Can you work these out from the model? Positions are in its coordinate system, mm. A direction names the side the tool comes from. Round coordinates to 2 decimals unless told otherwise and drop trailing zeros. Loops run counter-clockwise (first coordinate to the right, second up) from the corner with the lowest first, then second, coordinate; pieces in that order, holes last. Notation, with made-up numbers: (-34.5, 82) -> (-14.5, 82) arc R17 ccw to (-14.5, 88) -> close; hole circle Ø4 at (-4.75, 8). An arc over 180 degrees is marked (long way). Use a Markdown table: item, result.
from build123d import *

# Parameters (mm, degrees)
SKETCH_1_R          = 2.5
EXTRUDE_1_DEPTH     = 180
SKETCH_2_R          = 82.250528809
CUT_EXTRUDE_1_DEPTH = 10
SKETCH_3_R          = 47.359827943
CUT_EXTRUDE_2_DEPTH = 200
SKETCH_4_R          = 50.055938799
CUT_EXTRUDE_3_DEPTH = 30
SKETCH_5_R          = 35.776746529
CUT_EXTRUDE_4_DEPTH = 40
SKETCH_1_3_R        = 2.5
EXTRUDE_2_DEPTH     = 200
SKETCH_6_R          = 45.508426161
CUT_EXTRUDE_5_DEPTH = 50
SKETCH_7_R          = 85.251485325
CUT_EXTRUDE_7_DEPTH = 20


with BuildPart() as part:
    # Sketch 1 → Extrude 1 (new, symmetric)
    with BuildSketch(Plane(origin=(0, 0, 0), x_dir=(1, 0, 0), z_dir=(0, 1, 0))):
        Polygon((-15, -3.15), (-12.5, -3.15), (-12.5, -5.15), (-7, -5.15), (-7, -3.15), (-4.5, -3.15), (-4.5, 3.15), (-7, 3.15), (-7, 5.15), (-12.5, 5.15), (-12.5, 3.15), (-15, 3.15), (-15, 15), (-3.15, 15), (-3.15, 12.5), (-5.15, 12.5), (-5.15, 7), (-3.15, 7), (-3.15, 4.5), (3.15, 4.5), (3.15, 7), (5.15, 7), (5.15, 12.5), (3.15, 12.5), (3.15, 15), (15, 15), (15, 3.15), (12.5, 3.15), (12.5, 5.15), (7, 5.15), (7, 3.15), (4.5, 3.15), (4.5, -3.15), (7, -3.15), (7, -5.15), (12.5, -5.15), (12.5, -3.15), (15, -3.15), (15, -15), (3.15, -15), (3.15, -12.5), (5.15, -12.5), (5.15, -7), (3.15, -7), (3.15, -4.5), (-3.15, -4.5), (-3.15, -7), (-5.15, -7), (-5.15, -12.5), (-3.15, -12.5), (-3.15, -15), (-15, -15), align=None)
        with Locations(Location((-9.75, -9.75, 0), (0, 0, 90))):
            Circle(SKETCH_1_R, mode=Mode.SUBTRACT)
        with Locations(Location((-9.75, 9.75, 0), (0, 0, 90))):
            Circle(SKETCH_1_R, mode=Mode.SUBTRACT)
        with Locations(Location((9.75, 9.75, 0), (0, 0, 90))):
            Circle(SKETCH_1_R, mode=Mode.SUBTRACT)
        with Locations(Location((9.75, -9.75, 0), (0, 0, 90))):
            Circle(SKETCH_1_R, mode=Mode.SUBTRACT)
    extrude(amount=EXTRUDE_1_DEPTH, both=True)

    # Sketch 2 → Cut-Extrude 1 (cut)
    with BuildSketch(Plane(origin=(0, 180, 0), x_dir=(1, 0, 0), z_dir=(0, 1, 0))):
        Circle(SKETCH_2_R)
    extrude(amount=-CUT_EXTRUDE_1_DEPTH, mode=Mode.SUBTRACT)

    # Sketch 3 → Cut-Extrude 2 (cut)
    with BuildSketch(Plane.XZ.offset(180)):
        with Locations((0.216432031, -1.772037256)):
            Circle(SKETCH_3_R)
    extrude(amount=-CUT_EXTRUDE_2_DEPTH, mode=Mode.SUBTRACT)

    # Sketch 4 → Cut-Extrude 3 (cut)
    with BuildSketch(Plane.XZ.offset(-20)):
        with Locations((-1.287426062, -1.543634952)):
            Circle(SKETCH_4_R)
    extrude(amount=-CUT_EXTRUDE_3_DEPTH, mode=Mode.SUBTRACT)

    # Sketch 5 → Cut-Extrude 4 (cut)
    with BuildSketch(Plane.XZ.offset(-50)):
        with Locations((-0.979370242, 0.864150214)):
            Circle(SKETCH_5_R)
    extrude(amount=-CUT_EXTRUDE_4_DEPTH, mode=Mode.SUBTRACT)

    # Sketch 1_3 → Extrude 2 (add)
    with BuildSketch(Plane(origin=(0, 0, 0), x_dir=(1, 0, 0), z_dir=(0, 1, 0))):
        Polygon((-15, -3.15), (-12.5, -3.15), (-12.5, -5.15), (-7, -5.15), (-7, -3.15), (-4.5, -3.15), (-4.5, 3.15), (-7, 3.15), (-7, 5.15), (-12.5, 5.15), (-12.5, 3.15), (-15, 3.15), (-15, 15), (-3.15, 15), (-3.15, 12.5), (-5.15, 12.5), (-5.15, 7), (-3.15, 7), (-3.15, 4.5), (3.15, 4.5), (3.15, 7), (5.15, 7), (5.15, 12.5), (3.15, 12.5), (3.15, 15), (15, 15), (15, 3.15), (12.5, 3.15), (12.5, 5.15), (7, 5.15), (7, 3.15), (4.5, 3.15), (4.5, -3.15), (7, -3.15), (7, -5.15), (12.5, -5.15), (12.5, -3.15), (15, -3.15), (15, -15), (3.15, -15), (3.15, -12.5), (5.15, -12.5), (5.15, -7), (3.15, -7), (3.15, -4.5), (-3.15, -4.5), (-3.15, -7), (-5.15, -7), (-5.15, -12.5), (-3.15, -12.5), (-3.15, -15), (-15, -15), align=None)
        with Locations(Location((-9.75, -9.75, 0), (0, 0, 90))):
            Circle(SKETCH_1_3_R, mode=Mode.SUBTRACT)
        with Locations(Location((-9.75, 9.75, 0), (0, 0, 90))):
            Circle(SKETCH_1_3_R, mode=Mode.SUBTRACT)
        with Locations(Location((9.75, 9.75, 0), (0, 0, 90))):
            Circle(SKETCH_1_3_R, mode=Mode.SUBTRACT)
        with Locations(Location((9.75, -9.75, 0), (0, 0, 90))):
            Circle(SKETCH_1_3_R, mode=Mode.SUBTRACT)
    extrude(amount=EXTRUDE_2_DEPTH)

    # Sketch 6 → Cut-Extrude 5 (cut)
    with BuildSketch(Plane(origin=(0, 200, 0), x_dir=(1, 0, 0), z_dir=(0, 1, 0))):
        with Locations((-0.666782572, 0.500086929)):
            Circle(SKETCH_6_R)
    extrude(amount=-CUT_EXTRUDE_5_DEPTH, mode=Mode.SUBTRACT)

    # Sketch 7 → Cut-Extrude 7 (cut)
    with BuildSketch(Plane(origin=(0, 150, 0), x_dir=(1, 0, 0), z_dir=(0, 1, 0))):
        with Locations((0, -1.241240206)):
            Circle(SKETCH_7_R)
    extrude(amount=-CUT_EXTRUDE_7_DEPTH, mode=Mode.SUBTRACT)


solid = part.part
1. Will this pin go through, and if not, where does the flat tip stop? pin 1 Ø8 at (y, z) = (80, -3) entering from +X.
Answer sheet:
| item | result |
|---|---|
| pin 1 | stops at x = 15 |
2. I want a section at D-D (z = -1.5). Please give me the cut outline in (x, y).
Answer sheet:
| item | result |
|---|---|
| outline | (-4.5, 0) -> (4.5, 0) -> (4.5, 130) -> (-4.5, 130) -> close |
3. I want a section at B-B (z = 9.75). Please give me the cut outline in (x, y), plus the area to 3 significant figures.
Answer sheet:
| item | result |
|---|---|
| outline | (-15, 0) -> (-12.25, 0) -> (-12.25, 130) -> (-15, 130) -> close; (-7.25, 0) -> (-5.15, 0) -> (-5.15, 130) -> (-7.25, 130) -> close; (5.15, 0) -> (7.25, 0) -> (7.25, 130) -> (5.15, 130) -> close; (12.25, 0) -> (15, 0) -> (15, 130) -> (12.25, 130) -> close |
| area | 1,260 mm² |
4. I want a section at A-A (x = -9.75). Please give me the cut outline in (y, z).
Answer sheet:
| item | result |
|---|---|
| outline | (0, -15) -> (130, -15) -> (130, -12.25) -> (0, -12.25) -> close; (0, -7.25) -> (130, -7.25) -> (130, -5.15) -> (0, -5.15) -> close; (0, 5.15) -> (130, 5.15) -> (130, 7.25) -> (0, 7.25) -> close; (0, 12.25) -> (130, 12.25) -> (130, 15) -> (0, 15) -> close |
5. If we mould it in two halves opening along X, with no side actions, what happens to faces 4 (the flat face through (0, 0, 0)), 5 (the flat face through (15, 64, 9)), 6 (the cylindrical face through (12.19, 64.09, -9.21))? For each: +X half, -X half, draft (parallel to the pull), parting line (faces both ways), or undercut.
Answer sheet:
| item | result |
|---|---|
| face 4 | draft |
| face 5 | +X half |
| face 6 | undercut |
6. I need wall thicknesses on line 1 (Z direction, x = -9.75, y = 40.5); line 2 (X direction, y = 29.5, z = 6.75). Which ranges of each line are inside material? Lowest first, please.
Answer sheet:
| item | result |
|---|---|
| line 1 | z = -15 to -12.25, -7.25 to -5.15, 5.15 to 7.25, 12.25 to 15 |
| line 2 | x = -15 to -3.15, 3.15 to 15 |
7. Which directions (+Z, -Z, +X, -X, +Y, -Y) give clear straight access to the entire face, cutting with the end or side of a thin tool? Please do faces 1 (the flat face through (-14, 64, -3.15)), 2 (the flat face through (14, 64, -3.15)), 3 (the flat face through (-3.15, 64, -6)).
Answer sheet:
| item | result |
|---|---|
| face 1 | -X, +Y, -Y |
| face 2 | +X, +Y, -Y |
| face 3 | -Z, +Y, -Y |
8. I want a section at C-C (y = 59). State how many separate pieces and enclosed holes the cut face has, plus the area to 3 significant figures.
Answer sheet:
| item | result |
|---|---|
| separate pieces | 1 |
| enclosed holes | 4 |
| area | 469 mm² |
